The drawing under review shows one solid part. Ordinate dimensions are in mm from its lowest x, y, z. A direction names the side the tool comes from. Coordinates: 2 decimals unless noted, no trailing zeros. Loops run counter-clockwise (first coordinate to the right, second up) from the corner with the lowest first, then second, coordinate; pieces in that order, holes last. Notation, with made-up numbers: M -27,66 L 3,66 A25 cw 3,87 Z; hole C 9.25,85 d3. An arc over 180 degrees is marked long. Put each result on its own line as item: value.
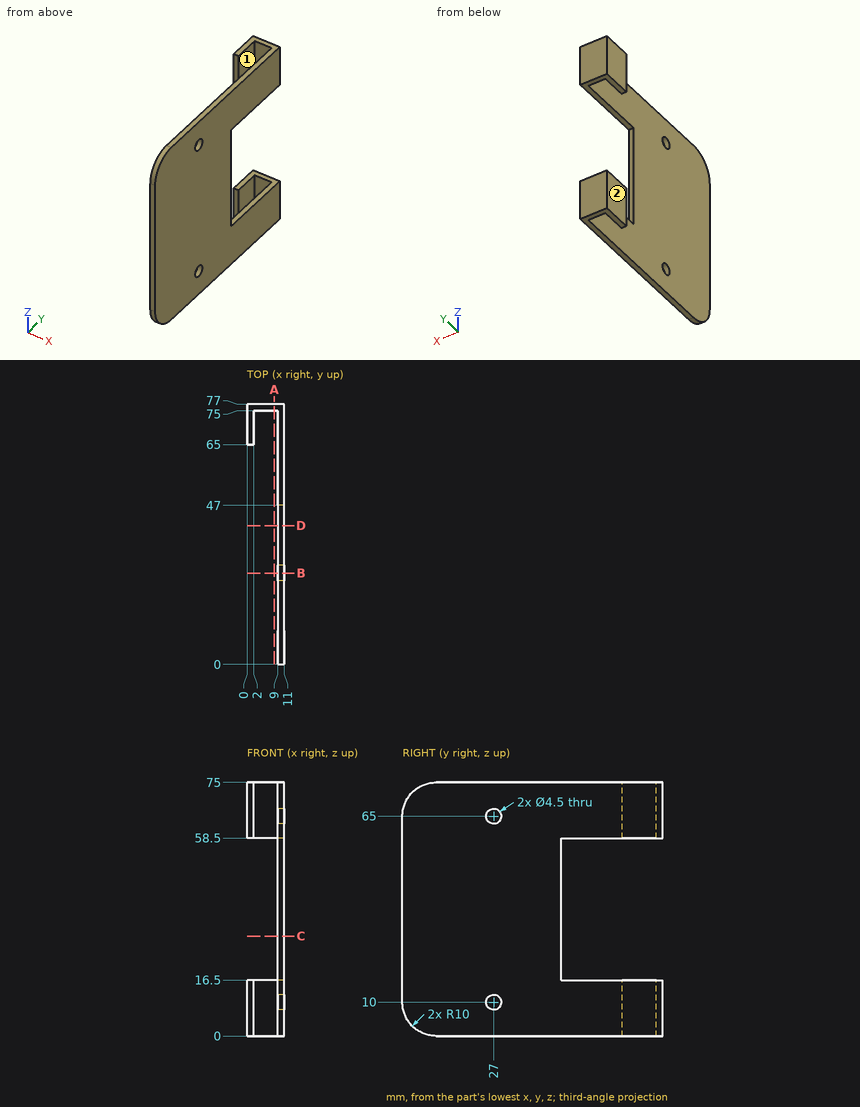
(1) Add section C-C (z = 29.5). Write out the cut boundary in (x, y), plus the area to 3 significant figures.
Determined:
outline: M 9,0 L 11,0 L 11,47 L 9,47 Z
area: 94.0 mm^2
(2) Tool access review of the marked faces 1 and 2: name each direction out of +Z, -Z, +X, -X, +Y, -Y from which nothing blocks a thin tool from reaching the whole face with its end or side.
Determined:
face 1: +Z, -Z, -Y
face 2: +Z, -Z, -X, +Y, -Y
(3) For pin 1 (2 mm diameter, centred on x = 1, z = 4.5, fed in from -Y); pin 2 (2 mm diameter, centred on x = 4.5, y = 67.5, fed in from -Z); pin 3 (2 mm diameter, centred on x = 10.5, z = 33, fed in from +Y); pin 4 (3 mm diameter, centred on y = 42.5, z = 58, fed in from -X), all flat-tipped, find the tip position at first contact; note any pin that passes through.
Determined:
pin 1: stops at y = 65
pin 2: passes through
pin 3: stops at y = 47
pin 4: stops at x = 9
(4) Add section A-A (x = 8). Write out the cut boundary in (y, z).
Determined:
outline: M 75,0 L 77,0 L 77,16.5 L 75,16.5 Z; M 75,58.5 L 77,58.5 L 77,75 L 75,75 Z
(5) Add section D-D (y = 41). Write out the cut boundary in (x, z), plus the area to 3 significant figures.
Determined:
outline: M 9,0 L 11,0 L 11,75 L 9,75 Z
area: 150 mm^2
(6) Add section B-B (y = 27). Write out the cut boundary in (x, z).
Determined:
outline: M 9,0 L 11,0 L 11,7.75 L 9,7.75 Z; M 9,12.25 L 11,12.25 L 11,62.75 L 9,62.75 Z; M 9,67.25 L 11,67.25 L 11,75 L 9,75 Z
(7) Wall thickness on line 1 along Z through (x, y) = (9.5, 27); line 2 along X through (y, z) = (65.5, 5); line 3 along Z through (x, y) = (1.75, 66): over which ranges is each line inside the solid? List them lowest first. Write a range as [from, to].
Determined:
line 1: z = [0, 7.75], [12.25, 62.75], [67.25, 75]
line 2: x = [0, 2], [9, 11]
line 3: z = [0, 16.5], [58.5, 75]
